```python
from build123d import *

# Parameters (mm, degrees)
PAD_DEPTH       = 3
PAD001_DEPTH    = 3
SKETCH002_W     = 209.08447
SKETCH002_H     = 4.18
PAD002_DEPTH    = 3
SKETCH003_W     = 26.3
SKETCH003_H     = 34.2
POCKET_DEPTH    = 3
SKETCH004_W     = 18
SKETCH004_H     = 25
POCKET001_DEPTH = 3
SKETCH005_W     = 14
SKETCH005_H     = 5
POCKET002_DEPTH = 6
SKETCH006_W     = 14
SKETCH006_H     = 3
POCKET003_DEPTH = 3
SKETCH007_W     = 8
SKETCH007_H     = 3
POCKET004_DEPTH = 3
SKETCH008_W     = 200
SKETCH008_H     = 4.4
PAD003_DEPTH    = 3
SKETCH009_R     = 0.82
POCKET005_DEPTH = 644.911736


with BuildPart() as part:
    # Sketch → Pad (new body)
    with BuildSketch(Plane.XY):
        with BuildLine():
            ThreePointArc((-100, 50), (-150, 0), (-100, -50))
            Line((-100, -50), (100, -50))
            ThreePointArc((100, -50), (150, 0), (100, 50))
            Line((-100, 50), (100, 50))
        make_face()
    extrude(amount=PAD_DEPTH)

    # Sketch001 (on Face6 of Pad) → Pad001 (join)
    with BuildSketch(Plane.XY.offset(3)):
        with BuildLine():
            ThreePointArc((-100, 50), (-150, 0), (-100, -50))
            Line((-100, -50), (100, -50))
            ThreePointArc((100, -50), (150, 0), (100, 50))
            Line((-100, 50), (100, 50))
        make_face()
        with BuildLine():
            ThreePointArc((-100, 5), (-105, 0), (-100, -5))
            Line((-100, -5), (100, -5))
            ThreePointArc((100, -5), (105, 0), (100, 5))
            Line((-100, 5), (100, 5))
        make_face(mode=Mode.SUBTRACT)
    extrude(amount=PAD001_DEPTH)

    # Sketch002 (on Face9 of Pad001) → Pad002 (join)
    with BuildSketch(Plane.XY.offset(6)):
        with BuildLine():
            ThreePointArc((-100, 50), (-150, 0), (-100, -50))
            Line((-100, -50), (100, -50))
            ThreePointArc((100, -50), (150, 0), (100, 50))
            Line((-100, 50), (100, 50))
        make_face()
        Rectangle(SKETCH002_W, SKETCH002_H, mode=Mode.SUBTRACT)
    extrude(amount=PAD002_DEPTH)

    # Sketch003 (on Face13 of Pad002) → Pocket (cut)
    with BuildSketch(Plane.XY.offset(9)):
        with Locations((0, -29.9)):
            Rectangle(SKETCH003_W, SKETCH003_H)
    extrude(amount=-POCKET_DEPTH, mode=Mode.SUBTRACT)

    # Sketch004 (on Face27 of Pocket) → Pocket001 (cut)
    with BuildSketch(Plane.XY.offset(6)):
        with Locations((0, -25.3)):
            Rectangle(SKETCH004_W, SKETCH004_H)
    extrude(amount=-POCKET001_DEPTH, mode=Mode.SUBTRACT)

    # Sketch005 (on Face13 of Pocket001) → Pocket002 (cut)
    with BuildSketch(Plane.XY.offset(9)):
        with Locations((0, -10.3)):
            Rectangle(SKETCH005_W, SKETCH005_H)
    extrude(amount=-POCKET002_DEPTH, mode=Mode.SUBTRACT)

    # Sketch006 (on Face23 of Pocket002) → Pocket003 (cut)
    with BuildSketch(Plane.XZ.offset(7.8)):
        with Locations((0, 4.5)):
            Rectangle(SKETCH006_W, SKETCH006_H)
    extrude(amount=-POCKET003_DEPTH, mode=Mode.SUBTRACT)

    # Sketch007 (on Face13 of Pocket003) → Pocket004 (cut)
    with BuildSketch(Plane.XY.offset(9)):
        with Locations((0, -48.5)):
            Rectangle(SKETCH007_W, SKETCH007_H)
    extrude(amount=-POCKET004_DEPTH, mode=Mode.SUBTRACT)

    # Sketch008 (on Face15 of Pocket004) → Pad003 (join)
    with BuildSketch(Plane.XY.offset(9)):
        with BuildLine():
            ThreePointArc((-100, 50), (-150, 0), (-100, -50))
            Line((-100, -50), (100, -50))
            ThreePointArc((100, -50), (150, 0), (100, 50))
            Line((-100, 50), (100, 50))
        make_face()
        Rectangle(SKETCH008_W, SKETCH008_H, mode=Mode.SUBTRACT)
    extrude(amount=PAD003_DEPTH)

    # Sketch009 (on Face4 of Pad003) → Pocket005 (cut, through all)
    with BuildSketch(Plane(origin=(0, 0, 0), x_dir=(1, 0, 0), z_dir=(0, 0, -1))):
        with Locations((-95, 35)):
            Circle(SKETCH009_R)
        with Locations((-95, -35)):
            Circle(SKETCH009_R)
    pocket005 = extrude(amount=-POCKET005_DEPTH, mode=Mode.SUBTRACT)

    # Mirrored: Pocket005 across Sketch009 V_Axis
    add(pocket005.mirror(Plane(origin=(0, 0, 0), x_dir=(0, 0, -1), z_dir=(1, 0, 0))), mode=Mode.SUBTRACT)


solid = part.part
```
Check sheet for the modelled part. Datum: model origin and axes. Units: mm. A direction names the side the tool comes from. Give positions to 0.01 mm unless a question says otherwise; leave off trailing zeros. Order: outer loops, then holes, each group sorted by start corner. A loop starts at its lowest first (then second) coordinate and runs counter-clockwise, first axis right, second up. Notation, with made-up numbers: M 32.5,83.25 L 55.5,83.25 A17 cw 55.5,116.25 Z; hole C 2.5,16 d1. An arc over 180 degrees is marked long. Answer in a Markdown table with one row per item. Add a question column.
Q1. Sectioned sample at A-A, the plane x = -69.5. Record the boundary of the cut face in (y, z), and give its area (3 significant figures).
Q2. Sectioned sample at C-C, the plane y = 31. Record the boundary of the cut face in (x, z), and give its area (3 significant figures).
Q3. Sectioned sample at B-B, the plane y = -26.5. Record the boundary of the cut face in (x, z), and give its area (3 significant figures).
Q4. Gauge pin test, flat ends, axial feed: pin 1 Ø21 at (x, y) = (-2.5, -32) entering from -Z; pin 2 Ø1.5 at (y, z) = (-20, 4) entering from -X; pin 3 Ø2.5 at (y, z) = (0.5, 8) entering from +X; pin 4 Ø5 at (y, z) = (5.5, 2) entering from +X. Record the tip position at first contact, or that the pin passes through.
Q5. Thickness scan on L1, parallel to Y at x = -95, z = 4; L2, parallel to Y at x = 95, z = 8.75; L3, parallel to X at y = 35, z = 9.5. Record the ranges inside material, lowest first.
Q6. Access from +Z, -Z, +X, -X, +Y, -Y to the whole of each face (thin tool, end or side, straight path). Record for faces 5 (the cylindrical face through (-149.988, 1.099, 5.916)), 6 (the flat face through (7, -10, 6)).
Q7. Release check for a two-part mould opening along Y. For faces 1 (the cylindrical face through (149.988, -1.099, 5.916)), 2 (the flat face through (-1, 50, 6)), 3 (the flat face through (0, -7, 3)), 4 (the flat face through (-2, 12, 12)) record: released by +Y, released by -Y, zero draft, split by the parting line, or undercut.
Verdict:
| question | item | result |
|---|---|---|
| 1 | outline | M -50,0 L 50,0 L 50,12 L 2.2,12 L 2.2,9 L 2.09,9 L 2.09,6 L 5,6 L 5,3 L -5,3 L -5,6 L -2.09,6 L -2.09,9 L -2.2,9 L -2.2,12 L -50,12 Z |
| 1 | area | 1,140 mm² |
| 2 | outline | M -139.23,0 L 139.23,0 L 139.23,12 L -139.23,12 Z |
| 2 | area | 3,340 mm² |
| 3 | outline | M -142.4,0 L 142.4,0 L 142.4,12 L -142.4,12 Z; hole M -13.15,6 L -9,6 L -9,3 L 9,3 L 9,6 L 13.15,6 L 13.15,9 L -13.15,9 Z |
| 3 | area | 3,280 mm² |
| 4 | pin 1 | z = 0 |
| 4 | pin 2 | x = -146.15 |
| 4 | pin 3 | x = 150 |
| 4 | pin 4 | x = 149.91 |
| 5 | L1 | -50 to -35.82, -34.18 to -5, 5 to 34.18, 35.82 to 50 |
| 5 | L2 | -50 to -35.82, -34.18 to -2.09, 2.09 to 34.18, 35.82 to 50 |
| 5 | L3 | -135.71 to -95.82, -94.18 to 94.18, 95.82 to 135.71 |
| 6 | face 5 | +Z, -Z, -X |
| 6 | face 6 | none |
| 7 | face 1 | split by the parting line |
| 7 | face 2 | released by +Y |
| 7 | face 3 | undercut |
| 7 | face 4 | zero draft |
